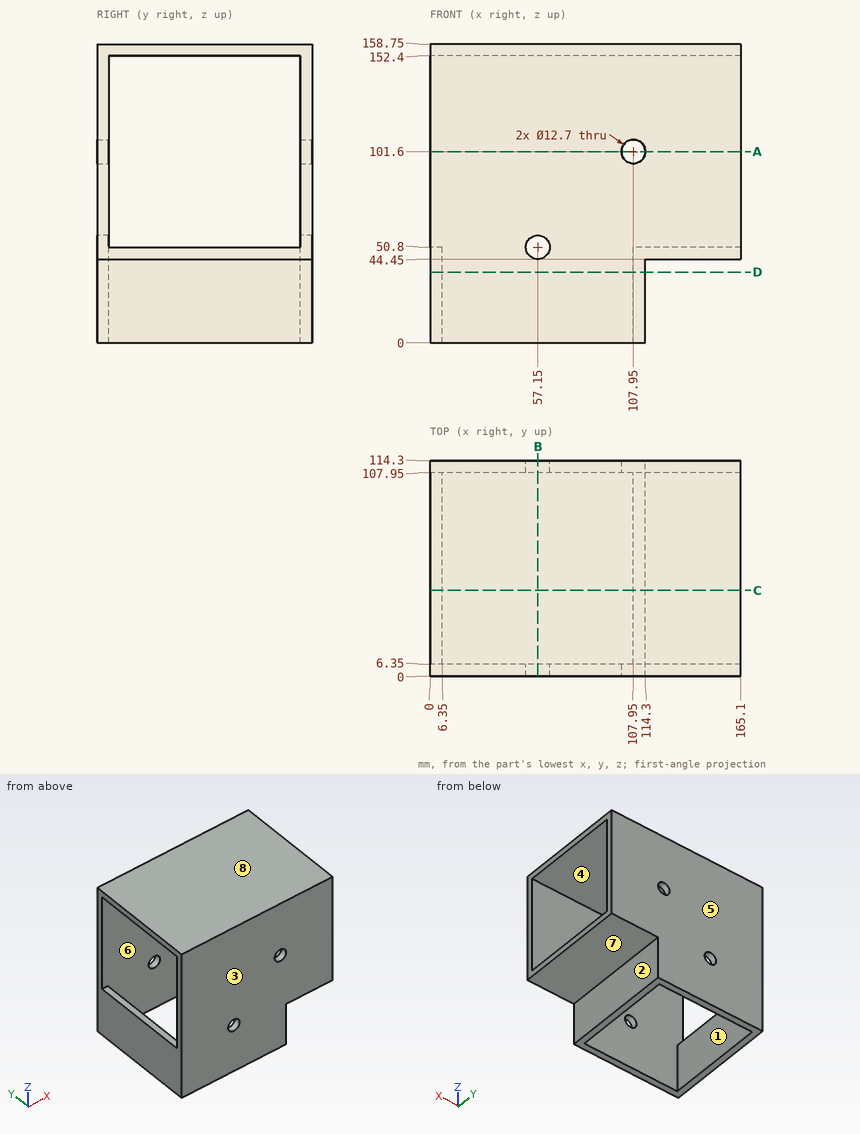
Print and shaded views of the part. All mm, measured from the part's lowest x, y and z. A direction names the side the tool comes from. Round coordinates to 2 decimals unless told otherwise and drop trailing zeros. Write each loop counter-clockwise with the first axis right and the second up, starting at its lowest first coordinate (ties: lowest second). Pieces come first, ordered by that corner, then holes. Notation, with made-up numbers: (8, 36) -> (58, 36) arc R28 ccw to (58, 56) -> close; hole circle Ø5 at (-14.5, 70). An arc over 180 degrees is marked (long way). Answer in a Markdown table with one row per item. Add a question column.
Item 1: Saw through at A-A, the plane z = 101.6. Write the cut outline in (x, y).
Item 2: Saw through at B-B, the plane x = 57.15. Write the cut outline in (y, z).
Item 3: Saw through at C-C, the plane y = 45.5. Write the cut outline in (x, z).
Item 4: Which spindle directions (+Z, -Z, +X, -X, +Y, -Y) get a long thin tool onto all of the face, cutting with end or side? Do the marked faces 4, 5, 6, 7 and 8. Say none if no direction does.
Item 5: Mould opens along X. For the marked faces 1, 2 and 3 say: pulls with the +X half, pulls with the -X half, needs draft (parallel to the pull), parting line crosses it, or undercut.
Item 6: Drop flat-ended pins along their axis: pin 1 Ø2 at (x, y) = (84.5, 13) entering from -Z; pin 2 Ø20.5 at (x, z) = (57.15, 50.8) entering from -Y; pin 3 Ø15 at (x, y) = (150, 81) entering from -Z; pin 4 Ø6 at (y, z) = (79.5, 27.5) entering from +X. Give the stop position or say it passes through.
Item 7: Saw through at D-D, the plane z = 37.5. Write the cut outline in (x, y), then the cut area to 3 significant figures.
Item 8: Drill centre lines: line 1 (Z direction, x = 108, y = 12); line 2 (Y direction, x = 86, z = 92.5). Where is each one in solid material? Low to high. Write a range as from..to.
Findings below:
| question | item | result |
|---|---|---|
| 1 | outline | (0, 0) -> (101.6, 0) -> (101.6, 6.35) -> (0, 6.35) -> close; (0, 107.95) -> (101.6, 107.95) -> (101.6, 114.3) -> (0, 114.3) -> close; (114.3, 0) -> (165.1, 0) -> (165.1, 6.35) -> (114.3, 6.35) -> close; (114.3, 107.95) -> (165.1, 107.95) -> (165.1, 114.3) -> (114.3, 114.3) -> close |
| 2 | outline | (0, 0) -> (6.35, 0) -> (6.35, 44.45) -> (0, 44.45) -> close; (0, 57.15) -> (6.35, 57.15) -> (6.35, 152.4) -> (107.95, 152.4) -> (107.95, 57.15) -> (114.3, 57.15) -> (114.3, 158.75) -> (0, 158.75) -> close; (107.95, 0) -> (114.3, 0) -> (114.3, 44.45) -> (107.95, 44.45) -> close |
| 3 | outline | (0, 0) -> (6.35, 0) -> (6.35, 50.8) -> (0, 50.8) -> close; (0, 152.4) -> (165.1, 152.4) -> (165.1, 158.75) -> (0, 158.75) -> close; (107.95, 0) -> (114.3, 0) -> (114.3, 44.45) -> (165.1, 44.45) -> (165.1, 50.8) -> (107.95, 50.8) -> close |
| 4 | face 4 | +X, -X |
| 4 | face 5 | +Z, -Z, +X, -X, +Y |
| 4 | face 6 | none |
| 4 | face 7 | -Z, +X, +Y, -Y |
| 4 | face 8 | +Z, +X, -X, +Y, -Y |
| 5 | face 1 | undercut |
| 5 | face 2 | pulls with the +X half |
| 5 | face 3 | needs draft |
| 6 | pin 1 | stops at z = 152.4 |
| 6 | pin 2 | stops at y = 0 |
| 6 | pin 3 | stops at z = 44.45 |
| 6 | pin 4 | stops at x = 114.3 |
| 7 | outline | (0, 0) -> (114.3, 0) -> (114.3, 114.3) -> (0, 114.3) -> close; hole (6.35, 6.35) -> (107.95, 6.35) -> (107.95, 107.95) -> (6.35, 107.95) -> close |
| 7 | area | 2,740 mm^2 |
| 8 | line 1 | z = 0..50.8, 152.4..158.75 |
| 8 | line 2 | y = 0..6.35, 107.95..114.3 |
